Autodesk Inventor part; units mm, degrees
ref_plane "YZ Plane" through (0, 0, 0) normal (1, 0, 0) x (0, 1, 0)
ref_plane "XZ Plane" through (0, 0, 0) normal (0, 1, 0) x (-1, 0, 0)
ref_plane "XY Plane" through (0, 0, 0) normal (0, 0, 1) x (1, 0, 0)
sketch "Sketch1" plane through (0, 0, 0) normal (0, 0, 1) x (1, 0, 0)
  line L0 (0, 0) -> (100, 0) construction
  line L1 (0, -10) -> (100, -10)
  line L2 (100, 10) -> (0, 10)
  arc A0 (0, 10) -> (0, -10) centre (0, 0) ccw
  arc A1 (100, -10) -> (100, 10) centre (100, 0) ccw
  line L3 (0, 0) -> (100, 0) construction
  circle A2 centre (0, 0) radius 4
  circle A3 centre (100, 0) radius 4
  circle A4 centre (50, 3.5) radius 1.5
  circle A5 centre (50, -3.5) radius 1.5
  circle A6 centre (107.5, 0) radius 1.5
  circle A7 centre (-7.5, 0) radius 1.5
  circle A8 centre (17, 0) radius 1.5
  circle A9 centre (83, 0) radius 1.5
  point P0 (50, 0)
  point P1 (50, 0)
  dimension "d0" = 100
  dimension "d1" = 0
  dimension "d2" = 20
  dimension "d3" = 8
  dimension "d4" = 8
  dimension "d5" = 3
  dimension "d6" = 3
  dimension "d7" = 3
  dimension "d8" = 3
  dimension "d9" = 0
  dimension "d10" = 7.5
  dimension "d11" = 0
  dimension "d12" = 7.5
  dimension "d13" = 3
  dimension "d14" = 3
  dimension "d15" = 3.5
  dimension "d16" = 3.5
  dimension "d17" = 17
  dimension "d18" = 17
  dimension "d19" = 0
  dimension "d20" = 0
extrude "Extrusion1" add sketch "Sketch1" along normal blind 3
sketch "Sketch2" plane through (0, 0, 3) normal (0, 0, 1) x (1, 0, 0)
  circle A0 centre (0, 0) radius 4
  circle A1 centre (100, 0) radius 4
  circle A2 centre (0, 0) radius 5.425
  circle A3 centre (100, 0) radius 5.425
  dimension "d23" = 10.85
  dimension "d24" = 10.85
extrude "Extrusion2" cut sketch "Sketch2" against normal blind 2 contours A0 | A1 | A2 | A3
sketch "Sketch3" plane through (0, 0, 3) normal (0, 0, 1) x (1, 0, 0)
  circle A0 centre (0, 0) radius 5.425
  circle A1 centre (100, 0) radius 5.425
  arc A2 (100, -10) -> (100, 10) centre (100, 0) ccw
  line L0 (100, 10) -> (0, 10)
  arc A3 (0, 10) -> (0, -10) centre (0, 0) ccw
  line L1 (0, -10) -> (100, -10)
  circle A4 centre (50, 3.5) radius 1.5
  circle A5 centre (50, -3.5) radius 1.5
  circle A6 centre (17, 0) radius 1.5
  circle A7 centre (83, 0) radius 1.5
  circle A8 centre (-7.5, 0) radius 1.5
  circle A9 centre (107.5, 0) radius 1.5
properties part number "Arm4_3D" material "Aluminum 6061, Welded"
Input: part model. Units: mm. Frame: model coordinates. A direction names the side the tool comes from. Give positions to 0.01 mm unless a question says otherwise; leave off trailing zeros. Order: outer loops, then holes, each group sorted by start corner. A loop starts at its lowest first (then second) coordinate and runs counter-clockwise, first axis right, second up. Notation, with made-up numbers: M 80,-16 L 139,-16 A24 cw 139,7 Z; hole C -18,-37 d1. An arc over 180 degrees is marked long. One line per question, with ' | ' between items. Start each with the question number.
1. Pull-direction query (X, two-part tool) for faces 1 (the face through (98, -4, 1)), 2 (the face through (110, 0, 1)), 3 (the face through (49, 0, 0)); classes: released by +X, released by -X, zero draft, split by the parting line, or undercut.
2. First-contact query: pin 1 Ø2.5 at (x, y) = (107.5, 0) entering from -Z; pin 2 Ø3.5 at (x, y) = (98, -1.5) entering from +Z. Flat tips, straight axial feed; report the tip coordinate or a pass-through.
3. Section query B-B (z = 1.55). Count the separate pieces of the cut face and the enclosed holes in it, and give its area (3 significant figures).
4. Section query C-C (x = 83). Return the cut outline in (y, z), and give its area (3 significant figures).
5. Material intervals for probe 1 along Y at (x, z) = (0, 2.5) (3 decimals); probe 2 along Y at (x, z) = (83, 1.3); probe 3 along Z at (x, y) = (-1, 5), sorted ascending. Write a range as [from, to].
6. Section query A-A (x = 50). Return the cut outline in (y, z), and give its area (3 significant figures).
7. Access query for faces 4 (the face through (-3.998, 3.666, 2.014)), 5 (the face through (-0.867, 3.905, 0.493)). Directions: +Z, -Z, +X, -X, +Y, -Y. A direction counts if a zero-diameter tool reaches every point of the face in a straight line with its end or side. Return the directions, or none.
Here are the results:
1) face 1: undercut | face 2: released by +X | face 3: zero draft
2) pin 1: through | pin 2: z = 1
3) separate pieces: 1 | enclosed holes: 8 | area: 2,090 mm²
4) outline: M -10,0 L -1.5,0 L -1.5,3 L -10,3 Z; M 1.5,0 L 10,0 L 10,3 L 1.5,3 Z | area: 51.0 mm²
5) probe 1: [-10, -5.425], [5.425, 10] | probe 2: [-10, -1.5], [1.5, 10] | probe 3: [0, 1]
6) outline: M -10,0 L -5,0 L -5,3 L -10,3 Z; M -2,0 L 2,0 L 2,3 L -2,3 Z; M 5,0 L 10,0 L 10,3 L 5,3 Z | area: 42.0 mm²
7) face 4: +Z | face 5: +Z, -Z
